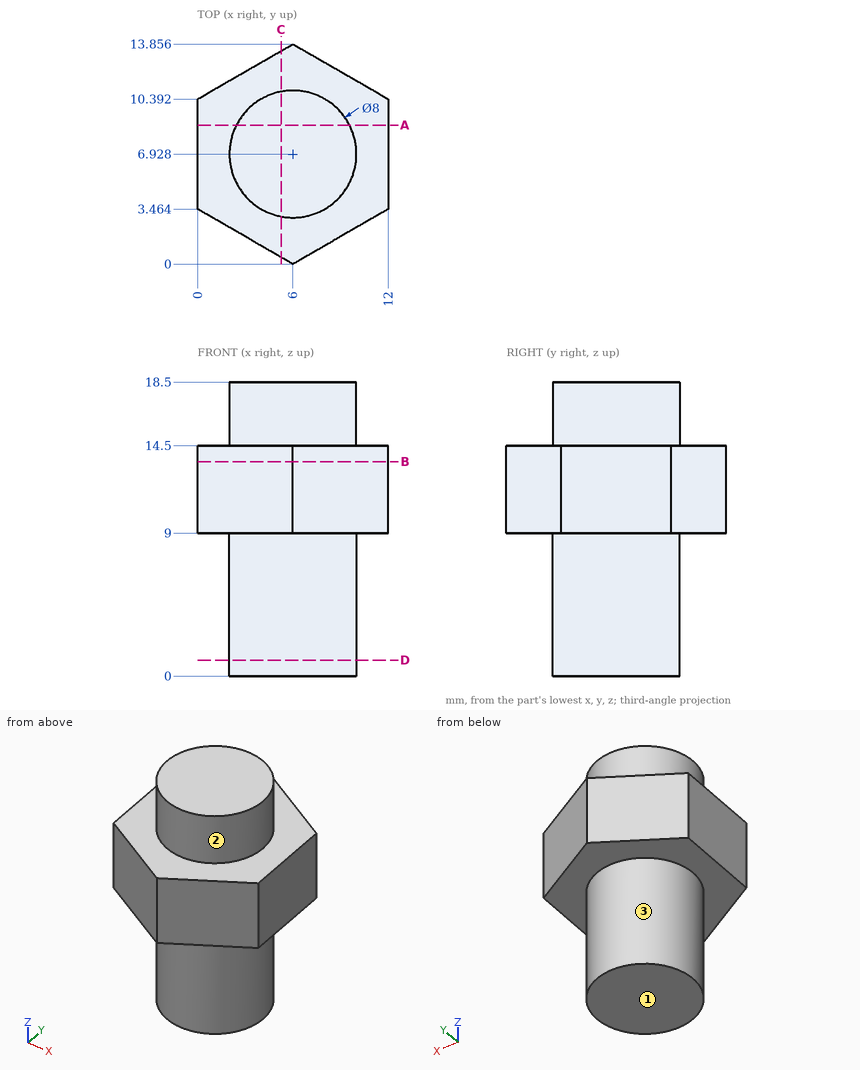
Part print with two shaded views. Sizes in mm from the minimum x, y, z corner. A direction names the side the tool comes from. Round coordinates to 2 decimals unless told otherwise and drop trailing zeros. Write each loop counter-clockwise with the first axis right and the second up, starting at its lowest first coordinate (ties: lowest second). Pieces come first, ordered by that corner, then holes. Notation, with made-up numbers: M -14,-25 L 23,-25 A18 cw 23,-17 Z; hole C 74.25,-25.5 d4. An arc over 180 degrees is marked long. Answer as CSV lines item,"result". Start each with the question number.
1) Band-saw the part on D-D (z = 1). List the corners of the cut face in (x, y).
2) Which spindle directions (+Z, -Z, +X, -X, +Y, -Y) get a long thin tool onto all of the face, cutting with end or side? Do the marked faces 1, 2 and 3. Say none if no direction does.
3) Band-saw the part on A-A (y = 8.75). List the corners of the cut face in (x, z), then the cut area to 3 significant figures.
4) Drill centre lines: L1, parallel to Z at x = 2.5, y = 3.75; L2, parallel to X at y = 6.75, z = 8.5; L3, parallel to Y at x = 6.25, z = 1.75. Where is each one in solid material? Low to high.
5) Band-saw the part on B-B (z = 13.5). List the corners of the cut face in (x, y).
6) Band-saw the part on C-C (x = 5.25). List the corners of the cut face in (y, z), then the cut area to 3 significant figures.
7) Drop flat-ended pins along their axis: pin 1 (3 mm diameter, centred on x = 2, y = 1.5, fed in from +Z); pin 2 (4 mm diameter, centred on x = 2.5, y = 4, fed in from -Z); pin 3 (5 mm diameter, centred on x = 8.5, z = 3, fed in from -Y); pin 4 (3 mm diameter, centred on y = 5.5, z = 3, fed in from +X). Give the stop position or say it passes through.
Worked out:
1,outline,"C 6,6.93 d8"
2,face 1,"-Z, +X, -X, +Y, -Y"
2,face 2,"+Z"
2,face 3,"-Z"
3,outline,"M 0,9 L 2.44,9 L 2.44,0 L 9.56,0 L 9.56,9 L 12,9 L 12,14.5 L 9.56,14.5 L 9.56,18.5 L 2.44,18.5 L 2.44,14.5 L 0,14.5 Z"
3,area,"159 mm²"
4,L1,"9 to 14.5"
4,L2,"2 to 10"
4,L3,"2.94 to 10.92"
5,outline,"M 0,3.46 L 6,0 L 12,3.46 L 12,10.39 L 6,13.86 L 0,10.39 Z"
6,outline,"M 0.43,9 L 3,9 L 3,0 L 10.86,0 L 10.86,9 L 13.42,9 L 13.42,14.5 L 10.86,14.5 L 10.86,18.5 L 3,18.5 L 3,14.5 L 0.43,14.5 Z"
6,area,"174 mm²"
7,pin 1,"z = 14.5"
7,pin 2,"z = 0"
7,pin 3,"y = 2.93"
7,pin 4,"x = 10"
